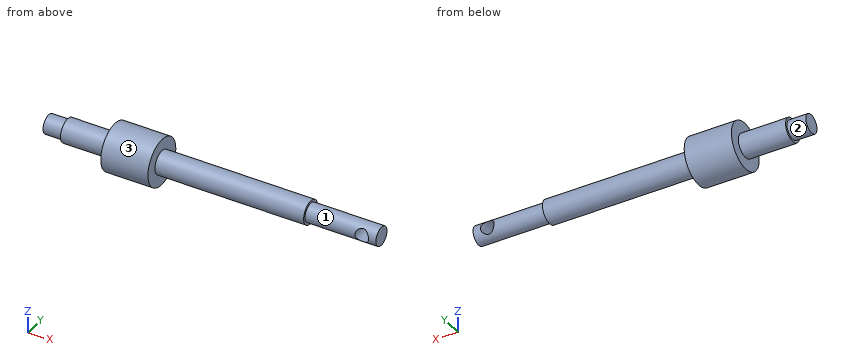
```python
from build123d import *

# Parameters (mm, degrees)
SKETCH_2_R          = 2
EXTRUDE_1_DEPTH     = 2
SKETCH_5_R          = 1.45
CUT_EXTRUDE_4_DEPTH = 5


with BuildPart() as part:
    # 草图1 → 旋转1 (revolve)
    with BuildSketch(Plane.XY):
        Polygon((-52.479220812, 2.5), (-52.479220812, 2), (-56.479220812, 2), (-56.479220812, 0), (12.020779188, 0), (12.020779188, 2), (-0.979220812, 2), (-0.979220812, 2.5), (-32.479220812, 2.5), (-32.479220812, 5), (-42.479220812, 5), (-42.479220812, 2.5), align=None)
    revolve(axis=Axis((-56.479220812, 0, 0), (1, 0, 0)))

    # 草图2 → 凸台-拉伸1 (add)
    with BuildSketch(Plane(origin=(12.020779188, 0, 0), x_dir=(0, 0, -1), z_dir=(1, 0, 0))):
        Circle(SKETCH_2_R)
    extrude(amount=EXTRUDE_1_DEPTH)

    # 草图5 → 切除-拉伸4 (cut, symmetric)
    with BuildSketch(Plane(origin=(0, 0, 0), x_dir=(1, 0, 0), z_dir=(0, 1, 0))):
        with Locations((11.020779188, 0)):
            Circle(SKETCH_5_R)
    extrude(amount=CUT_EXTRUDE_4_DEPTH, both=True, mode=Mode.SUBTRACT)


solid = part.part
```
Here's how the part is built. I have some questions about the finished solid (model axes, mm). Face numbers are marked on the shaded views. A direction names the side the tool comes from. Give positions to 0.01 mm unless a question says otherwise; leave off trailing zeros. Order: outer loops, then holes, each group sorted by start corner. A loop starts at its lowest first (then second) coordinate and runs counter-clockwise, first axis right, second up. Notation, with made-up numbers: (4, 4.25) - (57, 4.25) arc R19 cw to (57, 41.25) - close; hole circle Ø3 at (23.25, 39). An arc over 180 degrees is marked (long way). Answer as a JSON object with one key per item and string values. Group by question number.
Item 1: If we section it at D-D on x = -23.5: Please give me the cut outline in (y, z).
Item 2: For P1, Ø2, axis at x = -49, y = 3, coming from the -Z side; P2, Ø1.7, axis at x = 11.02, z = 0, coming from the +Y side; P3, Ø5, axis at x = -17, z = 2, coming from the -Y side; P4, Ø1, axis at y = 1, z = -3, coming from the +X side, each with a flat end and sliding along its axis, tell me the tip position at first contact or that it passes through.
Item 3: If we section it at B-B on y = 0: Please give me the cut outline in (x, z), and give its area (3 significant figures).
Item 4: Which directions (+Z, -Z, +X, -X, +Y, -Y) give clear straight access to the entire face, cutting with the end or side of a thin tool? Please do the marked faces 1, 2 and 3.
Item 5: If we section it at C-C on x = 6.5: Please give me the cut outline in (y, z), and give its area (3 significant figures).
Item 6: Please list where these lines run through material, in increasing order: probe 1 along X at (y, z) = (0.8, 0); probe 2 along X at (y, z) = (-3.5, -2); probe 3 along X at (y, z) = (-1.5, -0.75).
Item 7: If we section it at A-A on z = 0: Please give me the cut outline in (x, y), and give its area (3 significant figures).
Result set:
{
 "1": {"outline": "circle Ø5 at (0, 0)"},
 "2": {"P1": "z = -1.5", "P2": "through", "P3": "y = -2.5", "P4": "x = -32.48"},
 "3": {"outline": "(-56.48, -2) - (-52.48, -2) - (-52.48, -2.5) - (-42.48, -2.5) - (-42.48, -5) - (-32.48, -5) - (-32.48, -2.5) - (-0.98, -2.5) - (-0.98, -2) - (14.02, -2) - (14.02, 2) - (-0.98, 2) - (-0.98, 2.5) - (-32.48, 2.5) - (-32.48, 5) - (-42.48, 5) - (-42.48, 2.5) - (-52.48, 2.5) - (-52.48, 2) - (-56.48, 2) - close; hole circle Ø2.9 at (11.02, 0)", "area": "377 mm²"},
 "4": {"face 1": "+X", "face 2": "-X", "face 3": "+X, -X"},
 "5": {"outline": "circle Ø4 at (0, 0)", "area": "12.6 mm²"},
 "6": {"probe 1": "-56.48 to 9.57, 12.47 to 14.02", "probe 2": "-42.48 to -32.48", "probe 3": "-56.48 to 9.78, 12.26 to 14.02"},
 "7": {"outline": "(-56.48, -2) - (-52.48, -2) - (-52.48, -2.5) - (-42.48, -2.5) - (-42.48, -5) - (-32.48, -5) - (-32.48, -2.5) - (-0.98, -2.5) - (-0.98, -2) - (9.57, -2) - (9.57, 2) - (-0.98, 2) - (-0.98, 2.5) - (-32.48, 2.5) - (-32.48, 5) - (-42.48, 5) - (-42.48, 2.5) - (-52.48, 2.5) - (-52.48, 2) - (-56.48, 2) - close; (12.47, -2) - (14.02, -2) - (14.02, 2) - (12.47, 2) - close", "area": "372 mm²"}
}
